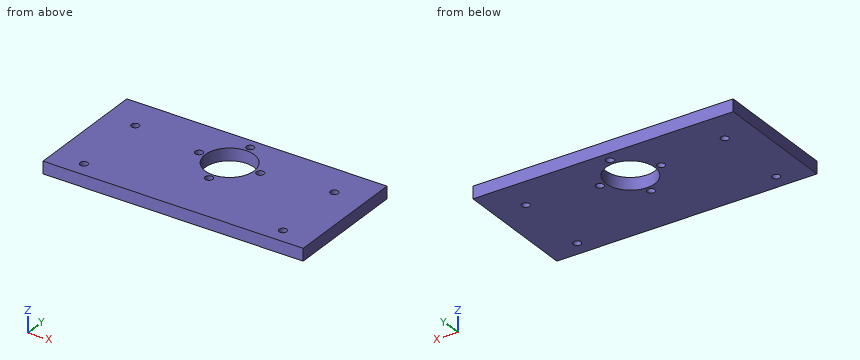
```python
from build123d import *

# Parameters (mm, degrees)
SKETCH1_W           = 170.035665534
SKETCH1_H           = 166.614386528
SKETCH1_R           = 16
BOSS_EXTRUDE1_DEPTH = 8
SKETCH2_R           = 2.5
SKETCH2_W           = 170.035665534
SKETCH2_H           = 56.759468899
SKETCH2_H_2         = 28.307193264
CUT_EXTRUDE1_DEPTH  = 120.298450693


with BuildPart() as part:
    # Sketch1 → Boss-Extrude1 (new body)
    with BuildSketch(Plane.XY):
        Rectangle(SKETCH1_W, SKETCH1_H)
        Circle(SKETCH1_R, mode=Mode.SUBTRACT)
    extrude(amount=BOSS_EXTRUDE1_DEPTH)

    # Sketch2 → Cut-Extrude1 (cut, through all)
    with BuildSketch(Plane.XY.offset(8)):
        with Locations((-65.017832767, 5)):
            Circle(SKETCH2_R)
        with Locations((-65.017832767, -45)):
            Circle(SKETCH2_R)
        with Locations((65.017832767, 5)):
            Circle(SKETCH2_R)
        with Locations((65.017832767, -45)):
            Circle(SKETCH2_R)
        with Locations((0, 20)):
            Circle(SKETCH2_R)
        with Locations((-20, 0)):
            Circle(SKETCH2_R)
        with Locations((0, -20)):
            Circle(SKETCH2_R)
        with Locations((20, 0)):
            Circle(SKETCH2_R)
        with Locations((0, 54.927458814)):
            Rectangle(SKETCH2_W, SKETCH2_H)
        with Locations((0, -69.153596632)):
            Rectangle(SKETCH2_W, SKETCH2_H_2)
    extrude(amount=-CUT_EXTRUDE1_DEPTH, mode=Mode.SUBTRACT)


solid = part.part
```
Read the model definition and answer for the solid it produces. Units are mm, in the model's axes. Give positions to 0.01 mm unless a question says otherwise; leave off trailing zeros. Write each loop counter-clockwise with the first axis right and the second up, starting at its lowest first coordinate (ties: lowest second). Pieces come first, ordered by that corner, then holes. Notation, with made-up numbers: (19, 61) -> (26, 61) arc R13 cw to (26, 67) -> close; hole circle Ø7 at (-15.5, 86). An arc over 180 degrees is marked (long way). Answer in a Markdown table with one row per item.
1) Section B-B on x = 20 is taken. Give the vertices of the cut face in (y, z), plus the area to 3 significant figures.
Results list:
| item | result |
|---|---|
| outline | (-55, 0) -> (-2.5, 0) -> (-2.5, 8) -> (-55, 8) -> close; (2.5, 0) -> (26.55, 0) -> (26.55, 8) -> (2.5, 8) -> close |
| area | 612 mm^2 |
2) Straight lines are drawn through the part: line 1 (Y direction, x = 0, z = 2); line 2 (Y direction, x = 20, z = 4.75); line 3 (X direction, y = -46.5, z = 3.25). For each, find the intervals that lie inside material, in ascending order. Write a range as [from, to].
Results list:
| item | result |
|---|---|
| line 1 | [-55, -22.5], [-17.5, -16], [16, 17.5], [22.5, 26.55] |
| line 2 | [-55, -2.5], [2.5, 26.55] |
| line 3 | [-85.02, -67.02], [-63.02, 63.02], [67.02, 85.02] |
3) Section C-C on y = 20 is taken. Give the vertices of the cut face in (x, z), plus the area to 3 significant figures.
Results list:
| item | result |
|---|---|
| outline | (-85.02, 0) -> (-2.5, 0) -> (-2.5, 8) -> (-85.02, 8) -> close; (2.5, 0) -> (85.02, 0) -> (85.02, 8) -> (2.5, 8) -> close |
| area | 1,320 mm^2 |
4) Section A-A on y = 0 is taken. Give the vertices of the cut face in (x, z).
Results list:
| item | result |
|---|---|
| outline | (-85.02, 0) -> (-22.5, 0) -> (-22.5, 8) -> (-85.02, 8) -> close; (-17.5, 0) -> (-16, 0) -> (-16, 8) -> (-17.5, 8) -> close; (16, 0) -> (17.5, 0) -> (17.5, 8) -> (16, 8) -> close; (22.5, 0) -> (85.02, 0) -> (85.02, 8) -> (22.5, 8) -> close |
5) Section D-D on x = 0 is taken. Give the vertices of the cut face in (y, z).
Results list:
| item | result |
|---|---|
| outline | (-55, 0) -> (-22.5, 0) -> (-22.5, 8) -> (-55, 8) -> close; (-17.5, 0) -> (-16, 0) -> (-16, 8) -> (-17.5, 8) -> close; (16, 0) -> (17.5, 0) -> (17.5, 8) -> (16, 8) -> close; (22.5, 0) -> (26.55, 0) -> (26.55, 8) -> (22.5, 8) -> close |
6) This flat-tipped pin is pushed along its axis until it touches: pin 1 Ø6.5 at (x, y) = (0, 20) entering from -Z. Where does it stop, or does it pass through?
Results list:
| item | result |
|---|---|
| pin 1 | z = 0 |
